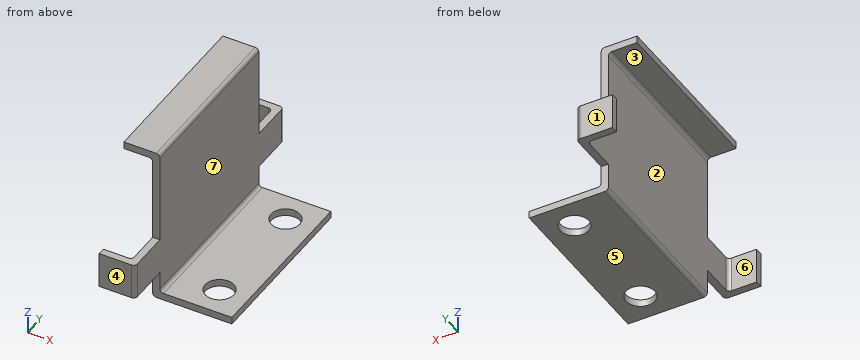
from build123d import *

# Parameters (mm, degrees)
F1_DEPTH = 24
F2_R     = 2
F3_DEPTH = 2
F4_W     = 6
F4_H     = 5
F5_DEPTH = 1
F6_W     = 1
F6_H     = 5
F7_DEPTH = 4
F8_R     = 0.5


with BuildPart() as f1:
    # F0 (on Front) → F1 (new body)
    with BuildSketch(Plane.XZ):
        Polygon((57.043818, 40.345872), (47.043818, 40.345872), (47.043818, 61.345872), (42.043818, 61.345872), (42.043818, 60.345872), (46.043818, 60.345872), (46.043818, 39.345872), (57.043818, 39.345872), align=None)
    extrude(amount=F1_DEPTH)

    # F2 (on face) → F3 (cut)
    with BuildSketch(Plane.XY.offset(40.345872)):
        with Locations((53.043818, -20)):
            Circle(F2_R)
        with Locations((53.043818, -4)):
            Circle(F2_R)
    extrude(amount=-F3_DEPTH, mode=Mode.SUBTRACT)

    # F4 (on face) → F5 (join)
    with BuildSketch(Plane.YZ.offset(47.043818)):
        with Locations((-27, 45.845872)):
            Rectangle(F4_W, F4_H)
        with Locations((3, 45.845872)):
            Rectangle(F4_W, F4_H)
    extrude(amount=-F5_DEPTH)

    # F6 (on face) → F7 (join)
    with BuildSketch(Plane(origin=(46.043818, 0, 0), x_dir=(0, -1, 0), z_dir=(-1, 0, 0))):
        with Locations((-5.5, 45.845872)):
            Rectangle(F6_W, F6_H)
        with Locations((29.5, 45.845872)):
            Rectangle(F6_W, F6_H)
    extrude(amount=F7_DEPTH)

    # F8
    f8_edges = [f1.edges().sort_by_distance(p)[0] for p in [
        (47.043818, -12, 40.345872),
        (46.043818, -12, 39.345872),
        (47.043818, -12, 61.345872),
        (46.043818, -12, 60.345872),
        (47.043818, -30, 45.845872),
        (46.043818, -29, 45.845872),
        (46.043818, 5, 45.845872),
        (47.043818, 6, 45.845872),
    ]]
    fillet(f8_edges, radius=F8_R)


solid = f1.part
Model file for the job. Use its own axes, mm. Face numbers are marked on the shaded views. A direction names the side the tool comes from. Give positions to 0.01 mm unless a question says otherwise; leave off trailing zeros. Order: outer loops, then holes, each group sorted by start corner. A loop starts at its lowest first (then second) coordinate and runs counter-clockwise, first axis right, second up. Notation, with made-up numbers: M -19.75,-13.5 L 13.25,-13.5 A24 ccw 13.25,24.5 Z; hole C 12,4.25 d3. An arc over 180 degrees is marked long. Put each result on its own line as item: value. Start each with the question number.
(1) Band-saw the part on A-A on x = 43.5. Give the cut face in (y, z).
(2) Band-saw the part on C-C on y = -11. Give the cut face in (x, z), then the cut area to 3 significant figures.
(3) Tool access for the marked faces 5, 6 and 7: list every direction of +Z, -Z, +X, -X, +Y, -Y with a clear straight run to the whole face (end or side of a thin tool).
(4) Band-saw the part on D-D on z = 42.25. Give the cut face in (x, y).
(5) Band-saw the part on B-B on y = -20. Give the cut face in (x, z), then the cut area to 3 significant figures.
(6) Pull direction Y, two halves, no side cores. Call the marked faces 1, 2, 3 and 4: released by +Y, released by -Y, zero draft, split by the parting line, or undercut.
(7) Pin check, flat tips, straight feed: pin 1 Ø5 at (x, y) = (53.04, -4) entering from +Z; pin 2 Ø4.5 at (x, z) = (51.5, 41) entering from +Y; pin 3 Ø3 at (x, z) = (52.5, 41) entering from -Y. Stop position of each tip, or through.
(8) Drill centre lines: L1, parallel to X at y = -5, z = 50.75; L2, parallel to Z at x = 56.5, y = -12.5; L3, parallel to Z at x = 44.5, y = -16.5. Where is each one in solid material? Low to high. Write a range as [from, to].
Results below:
1. outline: M -30,43.35 L -29,43.35 L -29,48.35 L -30,48.35 Z; M -24,60.35 L 0,60.35 L 0,61.35 L -24,61.35 Z; M 5,43.35 L 6,43.35 L 6,48.35 L 5,48.35 Z
2. outline: M 42.04,60.35 L 45.54,60.35 A0.5 cw 46.04,59.85 L 46.04,39.85 A0.5 ccw 46.54,39.35 L 57.04,39.35 L 57.04,40.35 L 47.54,40.35 A0.5 cw 47.04,40.85 L 47.04,60.85 A0.5 ccw 46.54,61.35 L 42.04,61.35 Z
2. area: 36.0 mm2
3. face 5: -Z, +X, -X, +Y, -Y
3. face 6: +Z, -Z, -X
3. face 7: +Z, +X, +Y, -Y
4. outline: M 46.04,-24 L 47.04,-24 L 47.04,0 L 46.04,0 Z
5. outline: M 42.04,60.35 L 45.54,60.35 A0.5 cw 46.04,59.85 L 46.04,39.85 A0.5 ccw 46.54,39.35 L 51.04,39.35 L 51.04,40.35 L 47.54,40.35 A0.5 cw 47.04,40.85 L 47.04,60.85 A0.5 ccw 46.54,61.35 L 42.04,61.35 Z; M 55.04,39.35 L 57.04,39.35 L 57.04,40.35 L 55.04,40.35 Z
5. area: 32.0 mm2
6. face 1: released by +Y
6. face 2: undercut
6. face 3: zero draft
6. face 4: released by -Y
7. pin 1: stops at z = 40.35
7. pin 2: stops at y = 0
7. pin 3: stops at y = -24
8. L1: x = [46.04, 47.04]
8. L2: z = [39.35, 40.35]
8. L3: z = [60.35, 61.35]
